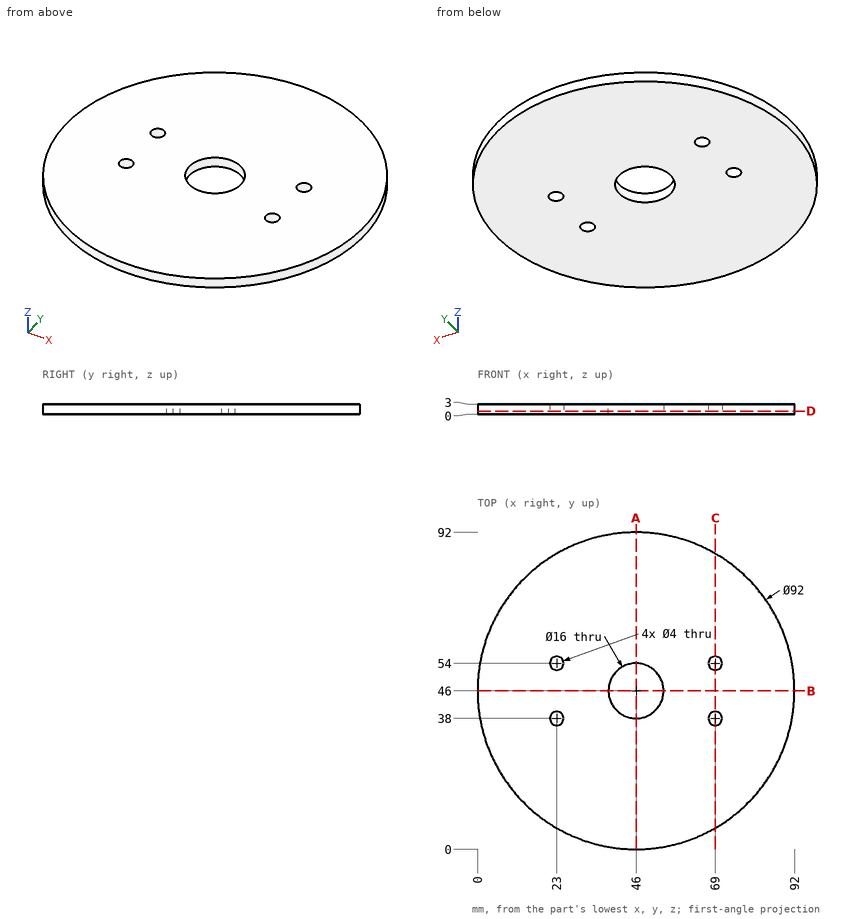
Study the drawing (mm; zero at the part's minimum x, y, z) and answer. Give positions to 0.01 mm unless a question says otherwise; leave off trailing zeros. Write each loop counter-clockwise with the first axis right and the second up, starting at its lowest first coordinate (ties: lowest second). Pieces come first, ordered by that corner, then holes. Notation, with made-up numbers: (84.25, 34) -> (95.25, 34) arc R19 cw to (95.25, 43) -> close; hole circle Ø8 at (25, 59). An arc over 180 degrees is marked (long way). Write item = value, one per line. Start each with the question number.
1) Straight lines are drawn through the part: line 1 along X through (y, z) = (55, 2.6); line 2 along Y through (x, z) = (23, 0.8); line 3 along Y through (x, z) = (41, 1.6) (3 decimals). For each, find the intervals that lie inside material, in ascending order.
2) The part is cut by section A-A, the plane x = 46. Determine the outline of the cut face in (y, z).
3) The part is cut by section C-C, the plane x = 69. Determine the outline of the cut face in (y, z), and give its area (3 significant figures).
4) The part is cut by section D-D, the plane z = 0.9. Determine the outline of the cut face in (x, y), and give its area (3 significant figures).
Solutions:
q1.line_1 = 0.89 to 21.27, 24.73 to 67.27, 70.73 to 91.11
q1.line_2 = 6.16 to 36, 40 to 52, 56 to 85.84
q1.line_3 = 0.273 to 39.755, 52.245 to 91.727
q2.outline = (0, 0) -> (38, 0) -> (38, 3) -> (0, 3) -> close; (54, 0) -> (92, 0) -> (92, 3) -> (54, 3) -> close
q3.outline = (6.16, 0) -> (36, 0) -> (36, 3) -> (6.16, 3) -> close; (40, 0) -> (52, 0) -> (52, 3) -> (40, 3) -> close; (56, 0) -> (85.84, 0) -> (85.84, 3) -> (56, 3) -> close
q3.area = 215 mm²
q4.outline = circle Ø92 at (46, 46); hole circle Ø4 at (23, 38); hole circle Ø4 at (23, 54); hole circle Ø16 at (46, 46); hole circle Ø4 at (69, 38); hole circle Ø4 at (69, 54)
q4.area = 6,400 mm²
